CAD build for the part. Positions are in the model's coordinates, mm. Coordinates: 2 decimals unless noted, no trailing zeros. Loops run counter-clockwise (first coordinate to the right, second up) from the corner with the lowest first, then second, coordinate; pieces in that order, holes last. Notation, with made-up numbers: (8, 37) -> (23, 37) arc R24 ccw to (23, 62) -> close; hole circle Ø6 at (-33, 85.25). An arc over 180 degrees is marked (long way). Return JSON: item names as keys, results as strings. Group by question number.
(1) Saw through at A-A on x = 0. Write the cut outline in (y, z), then the cut area to 3 significant figures.
(2) Mould opens along Y. For faces 1 (the face through (0, 20, 1)), 2 (the face through (0, -20, 1)), 3 (the face through (-5.158, -3.955, 1.014)), 4 (the face through (15, 0, 1)) say: pulls with the +Y half, pulls with the -Y half, needs draft (parallel to the pull), parting line crosses it, or undercut.
(3) Flat gauge pins, fed straight in: pin 1 Ø1.5 at (x, y) = (-9, 14) entering from -Z; pin 2 Ø3.5 at (x, y) = (11, 11) entering from +Z. Where does each tip first touch, or does it go through?
(4) Saw through at C-C on y = 12.5. Write the cut outline in (x, z).
(5) Saw through at B-B on z = 0.95. Write the cut outline in (x, y), then the cut area to 3 significant figures.
(6) Probe L1, parallel to Y at x = 11, z = 1.55; L2, parallel to X at y = 11, z = 1.55; L3, parallel to X at y = -10, z = 1.25. List the from-to ranges inside material, lowest first.
```python
from build123d import *

# Parameters (mm, degrees)
EXTRUDE_1_DEPTH     = 2
SKETCH_2_R          = 6.5
CUT_EXTRUDE_1_DEPTH = 2
SKETCH_5_W          = 30
SKETCH_5_H          = 2
EXTRUDE_4_DEPTH     = 5
SKETCH_6_W          = 30
SKETCH_6_H          = 2
EXTRUDE_5_DEPTH     = 5


with BuildPart() as part:
    # ｽｹｯﾁ1 → ﾎﾞｽ - 押し出し1 (new body)
    with BuildSketch(Plane.XY):
        with BuildLine():
            Line((11, 15), (-11, 15))
            Line((-11, 15), (-11, 13.1))
            ThreePointArc((-11, 13.1), (-9.51507576, 12.48492424), (-8.9, 11))
            ThreePointArc((-8.9, 11), (-11, 8.9), (-13.1, 11))
            Line((-13.1, 11), (-15, 11))
            Line((-15, 11), (-15, -11))
            Line((-15, -11), (-13.1, -11))
            ThreePointArc((-13.1, -11), (-11, -8.9), (-8.9, -11))
            ThreePointArc((-8.9, -11), (-9.51507576, -12.48492424), (-11, -13.1))
            Line((-11, -13.1), (-11, -15))
            Line((-11, -15), (11, -15))
            Line((11, -15), (11, -13.1))
            ThreePointArc((11, -13.1), (9.51507576, -9.51507576), (13.1, -11))
            Line((13.1, -11), (15, -11))
            Line((15, -11), (15, 11))
            Line((15, 11), (13.1, 11))
            ThreePointArc((13.1, 11), (9.51507576, 9.51507576), (11, 13.1))
            Line((11, 13.1), (11, 15))
        make_face()
        with BuildLine():
            Line((15, -15), (15, -11))
            Line((15, -11), (13.1, -11))
            ThreePointArc((13.1, -11), (12.48492424, -12.48492424), (11, -13.1))
            Line((11, -13.1), (11, -15))
            Line((11, -15), (15, -15))
        make_face()
        with BuildLine():
            Line((-13.1, -11), (-15, -11))
            Line((-15, -11), (-15, -15))
            Line((-15, -15), (-11, -15))
            Line((-11, -15), (-11, -13.1))
            ThreePointArc((-11, -13.1), (-12.48492424, -12.48492424), (-13.1, -11))
        make_face()
        with BuildLine():
            Line((-11, 15), (-15, 15))
            Line((-15, 15), (-15, 11))
            Line((-15, 11), (-13.1, 11))
            ThreePointArc((-13.1, 11), (-12.48492424, 12.48492424), (-11, 13.1))
            Line((-11, 13.1), (-11, 15))
        make_face()
        with BuildLine():
            Line((15, 15), (11, 15))
            Line((11, 15), (11, 13.1))
            ThreePointArc((11, 13.1), (12.48492424, 12.48492424), (13.1, 11))
            Line((13.1, 11), (15, 11))
            Line((15, 11), (15, 15))
        make_face()
    extrude(amount=EXTRUDE_1_DEPTH)

    # ｽｹｯﾁ2 → ｶｯﾄ - 押し出し1 (cut)
    with BuildSketch(Plane.XY.offset(2)):
        Circle(SKETCH_2_R)
    extrude(amount=-CUT_EXTRUDE_1_DEPTH, mode=Mode.SUBTRACT)

    # ｽｹｯﾁ5 → ﾎﾞｽ - 押し出し4 (add)
    with BuildSketch(Plane(origin=(0, 15, 0), x_dir=(1, 0, 0), z_dir=(0, 1, 0))):
        with Locations((0, -1)):
            Rectangle(SKETCH_5_W, SKETCH_5_H)
    extrude(amount=EXTRUDE_4_DEPTH)

    # ｽｹｯﾁ6 → ﾎﾞｽ - 押し出し5 (add)
    with BuildSketch(Plane(origin=(0, -15, 0), x_dir=(-1, 0, 0), z_dir=(0, -1, 0))):
        with Locations((0, -1)):
            Rectangle(SKETCH_6_W, SKETCH_6_H)
    extrude(amount=EXTRUDE_5_DEPTH)


solid = part.part
```
Geometry results:
{
 "1": {"outline": "(-20, 0) -> (-6.5, 0) -> (-6.5, 2) -> (-20, 2) -> close; (6.5, 0) -> (20, 0) -> (20, 2) -> (6.5, 2) -> close", "area": "54.0 mm²"},
 "2": {"face 1": "pulls with the +Y half", "face 2": "pulls with the -Y half", "face 3": "undercut", "face 4": "needs draft"},
 "3": {"pin 1": "z = 0", "pin 2": "through"},
 "4": {"outline": "(-15, 0) -> (-12.47, 0) -> (-12.47, 2) -> (-15, 2) -> close; (-9.53, 0) -> (9.53, 0) -> (9.53, 2) -> (-9.53, 2) -> close; (12.47, 0) -> (15, 0) -> (15, 2) -> (12.47, 2) -> close"},
 "5": {"outline": "(-15, -20) -> (15, -20) -> (15, 20) -> (-15, 20) -> close; hole circle Ø4.2 at (-11, -11); hole circle Ø4.2 at (-11, 11); hole circle Ø13 at (0, 0); hole circle Ø4.2 at (11, -11); hole circle Ø4.2 at (11, 11)", "area": "1,010 mm²"},
 "6": {"L1": "-20 to -13.1, -8.9 to 8.9, 13.1 to 20", "L2": "-15 to -13.1, -8.9 to 8.9, 13.1 to 15", "L3": "-15 to -12.85, -9.15 to 9.15, 12.85 to 15"}
}
